The model under review builds one solid part; all positions refer to its coordinate system, in mm. A direction names the side the tool comes from. Round coordinates to 2 decimals unless told otherwise and drop trailing zeros. Put each result on its own line as item: value. Start each with the question number.
from build123d import *

# Parameters (mm, degrees)
SKETCH1_R           = 8.025
BOSS_EXTRUDE1_DEPTH = 16
CUT_EXTRUDE1_START  = -8.55
SKETCH2_R           = 8.025
CUT_EXTRUDE1_DEPTH  = 7.35
SKETCH3_R           = 2.475
CUT_EXTRUDE2_DEPTH  = 20.616351598
CIRPATTERN1_COUNT   = 2
CIRPATTERN1_ANGLE   = 90


# Read off the part's stored shape, not the designer's step: M3x0.5 Tapped Hole1
with BuildPart() as part:
    # Sketch1 → Boss-Extrude1 (new body)
    with BuildSketch(Plane(origin=(0, 0, 0), x_dir=(1, 0, 0), z_dir=(0, 1, 0))):
        with Locations(Location((0, 0, 0), (0, 0, 270))):
            Circle(SKETCH1_R)
    extrude(amount=BOSS_EXTRUDE1_DEPTH)

    # Sketch2 → Cut-Extrude1 (cut)
    with BuildSketch(Plane(origin=(0, 16, 0), x_dir=(1, 0, 0), z_dir=(0, 1, 0)).offset(CUT_EXTRUDE1_START)):
        with Locations(Location((0, 0, 0), (0, 0, 270))):
            Circle(SKETCH2_R)
        with BuildLine():
            Line((0.223750509, 5.986515514), (0.617084741, 5.197309317))
            ThreePointArc((0.617084741, 5.197309317), (0.801726633, 5.061902746), (1.01917444, 5.133624565))
            Line((1.01917444, 5.133624565), (1.637135651, 5.762657299))
            ThreePointArc((1.637135651, 5.762657299), (1.756034951, 5.830288043), (1.892729091, 5.825221162))
            ThreePointArc((1.892729091, 5.825221162), (2.00629521, 5.748973556), (2.06273441, 5.62437188))
            Line((2.06273441, 5.62437188), (2.192939368, 4.752245221))
            ThreePointArc((2.192939368, 4.752245221), (2.326701311, 4.566408436), (2.555669726, 4.567424872))
            Line((2.555669726, 4.567424872), (3.337767568, 4.974710037))
            ThreePointArc((3.337767568, 4.974710037), (3.471746571, 5.002288793), (3.60018467, 4.955229091))
            ThreePointArc((3.60018467, 4.955229091), (3.684630662, 4.847619447), (3.699803496, 4.711675538))
            Line((3.699803496, 4.711675538), (3.55413381, 3.841998252))
            ThreePointArc((3.55413381, 3.841998252), (3.623922254, 3.623922254), (3.841998252, 3.55413381))
            Line((3.841998252, 3.55413381), (4.711675538, 3.699803496))
            ThreePointArc((4.711675538, 3.699803496), (4.847619447, 3.684630662), (4.955229091, 3.60018467))
            ThreePointArc((4.955229091, 3.60018467), (5.002288793, 3.471746571), (4.974710037, 3.337767568))
            Line((4.974710037, 3.337767568), (4.567424872, 2.555669726))
            ThreePointArc((4.567424872, 2.555669726), (4.566408436, 2.326701311), (4.752245221, 2.192939368))
            Line((4.752245221, 2.192939368), (5.62437188, 2.06273441))
            ThreePointArc((5.62437188, 2.06273441), (5.748973556, 2.00629521), (5.825221162, 1.892729091))
            ThreePointArc((5.825221162, 1.892729091), (5.830288043, 1.756034951), (5.762657299, 1.637135651))
            Line((5.762657299, 1.637135651), (5.133624565, 1.01917444))
            ThreePointArc((5.133624565, 1.01917444), (5.061902746, 0.801726633), (5.197309317, 0.617084741))
            Line((5.197309317, 0.617084741), (5.986515514, 0.223750509))
            ThreePointArc((5.986515514, 0.223750509), (6.087578078, 0.131569604), (6.125, 0))
            ThreePointArc((6.125, 0), (6.087578078, -0.131569604), (5.986515514, -0.223750509))
            Line((5.986515514, -0.223750509), (5.197309317, -0.617084741))
            ThreePointArc((5.197309317, -0.617084741), (5.061902746, -0.801726633), (5.133624565, -1.01917444))
            Line((5.133624565, -1.01917444), (5.762657299, -1.637135651))
            ThreePointArc((5.762657299, -1.637135651), (5.830288043, -1.756034951), (5.825221162, -1.892729091))
            ThreePointArc((5.825221162, -1.892729091), (5.748973556, -2.00629521), (5.62437188, -2.06273441))
            Line((5.62437188, -2.06273441), (4.752245221, -2.192939368))
            ThreePointArc((4.752245221, -2.192939368), (4.566408436, -2.326701311), (4.567424872, -2.555669726))
            Line((4.567424872, -2.555669726), (4.974710037, -3.337767568))
            ThreePointArc((4.974710037, -3.337767568), (5.002288793, -3.471746571), (4.955229091, -3.60018467))
            ThreePointArc((4.955229091, -3.60018467), (4.847619447, -3.684630662), (4.711675538, -3.699803496))
            Line((4.711675538, -3.699803496), (3.841998252, -3.55413381))
            ThreePointArc((3.841998252, -3.55413381), (3.623922254, -3.623922254), (3.55413381, -3.841998252))
            Line((3.55413381, -3.841998252), (3.699803496, -4.711675538))
            ThreePointArc((3.699803496, -4.711675538), (3.684630662, -4.847619447), (3.60018467, -4.955229091))
            ThreePointArc((3.60018467, -4.955229091), (3.471746571, -5.002288793), (3.337767568, -4.974710037))
            Line((3.337767568, -4.974710037), (2.555669726, -4.567424872))
            ThreePointArc((2.555669726, -4.567424872), (2.326701311, -4.566408436), (2.192939368, -4.752245221))
            Line((2.192939368, -4.752245221), (2.06273441, -5.62437188))
            ThreePointArc((2.06273441, -5.62437188), (2.00629521, -5.748973556), (1.892729091, -5.825221162))
            ThreePointArc((1.892729091, -5.825221162), (1.756034951, -5.830288043), (1.637135651, -5.762657299))
            Line((1.637135651, -5.762657299), (1.01917444, -5.133624565))
            ThreePointArc((1.01917444, -5.133624565), (0.801726633, -5.061902746), (0.617084741, -5.197309317))
            Line((0.617084741, -5.197309317), (0.223750509, -5.986515514))
            ThreePointArc((0.223750509, -5.986515514), (0.131569604, -6.087578078), (0, -6.125))
            ThreePointArc((0, -6.125), (-0.131569604, -6.087578078), (-0.223750509, -5.986515514))
            Line((-0.223750509, -5.986515514), (-0.617084741, -5.197309317))
            ThreePointArc((-0.617084741, -5.197309317), (-0.801726633, -5.061902746), (-1.01917444, -5.133624565))
            Line((-1.01917444, -5.133624565), (-1.637135651, -5.762657299))
            ThreePointArc((-1.637135651, -5.762657299), (-1.756034951, -5.830288043), (-1.892729091, -5.825221162))
            ThreePointArc((-1.892729091, -5.825221162), (-2.00629521, -5.748973556), (-2.06273441, -5.62437188))
            Line((-2.06273441, -5.62437188), (-2.192939368, -4.752245221))
            ThreePointArc((-2.192939368, -4.752245221), (-2.326701311, -4.566408436), (-2.555669726, -4.567424872))
            Line((-2.555669726, -4.567424872), (-3.337767568, -4.974710037))
            ThreePointArc((-3.337767568, -4.974710037), (-3.471746571, -5.002288793), (-3.60018467, -4.955229091))
            ThreePointArc((-3.60018467, -4.955229091), (-3.684630662, -4.847619447), (-3.699803496, -4.711675538))
            Line((-3.699803496, -4.711675538), (-3.55413381, -3.841998252))
            ThreePointArc((-3.55413381, -3.841998252), (-3.623922254, -3.623922254), (-3.841998252, -3.55413381))
            Line((-3.841998252, -3.55413381), (-4.711675538, -3.699803496))
            ThreePointArc((-4.711675538, -3.699803496), (-4.847619447, -3.684630662), (-4.955229091, -3.60018467))
            ThreePointArc((-4.955229091, -3.60018467), (-5.002288793, -3.471746571), (-4.974710037, -3.337767568))
            Line((-4.974710037, -3.337767568), (-4.567424872, -2.555669726))
            ThreePointArc((-4.567424872, -2.555669726), (-4.566408436, -2.326701311), (-4.752245221, -2.192939368))
            Line((-4.752245221, -2.192939368), (-5.62437188, -2.06273441))
            ThreePointArc((-5.62437188, -2.06273441), (-5.748973556, -2.00629521), (-5.825221162, -1.892729091))
            ThreePointArc((-5.825221162, -1.892729091), (-5.830288043, -1.756034951), (-5.762657299, -1.637135651))
            Line((-5.762657299, -1.637135651), (-5.133624565, -1.01917444))
            ThreePointArc((-5.133624565, -1.01917444), (-5.061902746, -0.801726633), (-5.197309317, -0.617084741))
            Line((-5.197309317, -0.617084741), (-5.986515514, -0.223750509))
            ThreePointArc((-5.986515514, -0.223750509), (-6.087578078, -0.131569604), (-6.125, 0))
            ThreePointArc((-6.125, 0), (-6.087578078, 0.131569604), (-5.986515514, 0.223750509))
            Line((-5.986515514, 0.223750509), (-5.197309317, 0.617084741))
            ThreePointArc((-5.197309317, 0.617084741), (-5.061902746, 0.801726633), (-5.133624565, 1.01917444))
            Line((-5.133624565, 1.01917444), (-5.762657299, 1.637135651))
            ThreePointArc((-5.762657299, 1.637135651), (-5.830288043, 1.756034951), (-5.825221162, 1.892729091))
            ThreePointArc((-5.825221162, 1.892729091), (-5.748973556, 2.00629521), (-5.62437188, 2.06273441))
            Line((-5.62437188, 2.06273441), (-4.752245221, 2.192939368))
            ThreePointArc((-4.752245221, 2.192939368), (-4.566408436, 2.326701311), (-4.567424872, 2.555669726))
            Line((-4.567424872, 2.555669726), (-4.974710037, 3.337767568))
            ThreePointArc((-4.974710037, 3.337767568), (-5.002288793, 3.471746571), (-4.955229091, 3.60018467))
            ThreePointArc((-4.955229091, 3.60018467), (-4.847619447, 3.684630662), (-4.711675538, 3.699803496))
            Line((-4.711675538, 3.699803496), (-3.841998252, 3.55413381))
            ThreePointArc((-3.841998252, 3.55413381), (-3.623922254, 3.623922254), (-3.55413381, 3.841998252))
            Line((-3.55413381, 3.841998252), (-3.699803496, 4.711675538))
            ThreePointArc((-3.699803496, 4.711675538), (-3.684630662, 4.847619447), (-3.60018467, 4.955229091))
            ThreePointArc((-3.60018467, 4.955229091), (-3.471746571, 5.002288793), (-3.337767568, 4.974710037))
            Line((-3.337767568, 4.974710037), (-2.555669726, 4.567424872))
            ThreePointArc((-2.555669726, 4.567424872), (-2.326701311, 4.566408436), (-2.192939368, 4.752245221))
            Line((-2.192939368, 4.752245221), (-2.06273441, 5.62437188))
            ThreePointArc((-2.06273441, 5.62437188), (-2.00629521, 5.748973556), (-1.892729091, 5.825221162))
            ThreePointArc((-1.892729091, 5.825221162), (-1.756034951, 5.830288043), (-1.637135651, 5.762657299))
            Line((-1.637135651, 5.762657299), (-1.01917444, 5.133624565))
            ThreePointArc((-1.01917444, 5.133624565), (-0.801726633, 5.061902746), (-0.617084741, 5.197309317))
            Line((-0.617084741, 5.197309317), (-0.223750509, 5.986515514))
            ThreePointArc((-0.223750509, 5.986515514), (-0.131569604, 6.087578078), (0, 6.125))
            ThreePointArc((0, 6.125), (0.131569604, 6.087578078), (0.223750509, 5.986515514))
        make_face(mode=Mode.SUBTRACT)
    extrude(amount=CUT_EXTRUDE1_DEPTH, mode=Mode.SUBTRACT)

    # Sketch3 → Cut-Extrude2 (cut, through all)
    with BuildSketch(Plane(origin=(0, 16, 0), x_dir=(1, 0, 0), z_dir=(0, 1, 0))):
        with Locations(Location((0, 0, 0), (0, 0, 270))):
            Circle(SKETCH3_R)
    extrude(amount=-CUT_EXTRUDE2_DEPTH, mode=Mode.SUBTRACT)

    # M3x0.5 Tapped Hole1 outline → M3x0.5 Tapped Hole1 (revolve, cut)
    with BuildSketch(Plane.XZ.offset(-3.725)):
        Polygon((2.000000319, 8.025000319), (0, 8.025000319), (0, 2.135986764), (1.25, 2.135986764), (1.25, 7.275), align=None)
    m3x0_5_tapped_hole1 = revolve(axis=Axis((0, 3.725, 0), (0, 0, 1)), mode=Mode.SUBTRACT)

    # CirPattern1: M3x0.5 Tapped Hole1 ×2 about axis
    cirpattern1_axis = Axis((0, 16, 0), (0, 1, 0))
    for i in range(1, CIRPATTERN1_COUNT):
        add(m3x0_5_tapped_hole1.rotate(cirpattern1_axis, i * CIRPATTERN1_ANGLE / (CIRPATTERN1_COUNT - 1)), mode=Mode.SUBTRACT)


solid = part.part
Q1. For faces 1 (the face through (5, 7.45, 3)), 2 (the face through (-2.127, 11.074, 5.194)), 3 (the face through (2.127, 11.074, -5.194)), 4 (the face through (3.628, 11.074, -4.283)), 5 (the face through (-5.18, 11.07, 2.13)), list the 3-axis set-ups (+Z, -Z, +X, -X, +Y, -Y) from which the entire face can be reached by the end or side of a thin tool; tool diameter is ignored.
Q2. Wall thickness on probe 1 along Y at (x, z) = (-2.25, -7); probe 2 along X at (y, z) = (1.25, 0) (3 decimals); probe 3 along Y at (x, z) = (3.7, 0) (3 decimals): over which ranges is each line inside the solid? List them lowest first. Write a range as [from, to].
Q3. Clearance check with flat-ended pins moving along their axes: pin 1 Ø3 at (y, z) = (3.725, 0) entering from +X (3 decimals); pin 2 Ø3 at (y, z) = (6.5, -5.5) entering from -X; pin 3 Ø8 at (y, z) = (10.5, -3) entering from +X; pin 4 Ø4 at (x, z) = (0, 0) entering from +Y. State where each tip first meets the part, or that it passes through.
Q4. Draft analysis for pull direction X (two halves, no side actions). For faces 6 (the face through (-2.13, 11.07, -5.18)), 7 (the face through (5.194, 11.074, 2.127)), 8 (the face through (4.742, 3.246, -1.155)), state which applies: +X half, -X half, draft (parallel to the pull), parting line (faces both ways), or undercut.
Calculated:
1. face 1: none
1. face 2: +Z
1. face 3: -Z
1. face 4: +X
1. face 5: -X
2. probe 1: y = [0, 7.45], [14.8, 16]
2. probe 2: x = [-8.025, -2.475], [2.475, 8.025]
2. probe 3: y = [0, 2.475], [4.975, 16]
3. pin 1: stops at x = 7.525
3. pin 2: stops at x = -6.96
3. pin 3: stops at x = 8.01
3. pin 4: passes through
4. face 6: undercut
4. face 7: +X half
4. face 8: draft
